from build123d import *

# Parameters (mm, degrees)
IZIM1_R                     = 27.1
Y_KSEKLIK_EKSTR_ZYON1_DEPTH = 3.3
IZIM3_R                     = 23.85
Y_KSEKLIK_EKSTR_ZYON2_DEPTH = 21.4
IZIM6_R                     = 20.35
KES_EKSTR_ZYON1_DEPTH       = 50


with BuildPart() as part:
    # Çizim1 → Yükseklik-Ekstrüzyon1 (new body)
    with BuildSketch(Plane.XY):
        Circle(IZIM1_R)
    extrude(amount=Y_KSEKLIK_EKSTR_ZYON1_DEPTH)

    # Çizim3 → Yükseklik-Ekstrüzyon2 (add)
    with BuildSketch(Plane.XY.offset(3.3)):
        Circle(IZIM3_R)
    extrude(amount=Y_KSEKLIK_EKSTR_ZYON2_DEPTH)

    # loft up to a face of the part (loft1)
    loft([Face(Wire([part.edges().sort_by_distance((-18.551226571, -19.755049803, 0))[0]])), Face(Wire([part.edges().sort_by_distance((-16.326448476, 17.385901764, 3.3))[0]]))])

    # Çizim5 → Kes-Döndür1 (revolve, cut)
    with BuildSketch(Plane(origin=(0, 0, 0), x_dir=(1, 0, 0), z_dir=(0, 1, 0))):
        Polygon((-27.1, 0), (-23.85, -3.3), (-27.1, -3.3), align=None)
    revolve(axis=Axis((0, 0, -4.734059464), (0, 0, 1)), mode=Mode.SUBTRACT)

    # Çizim6 → Kes-Ekstrüzyon1 (cut)
    with BuildSketch(Plane.XY.offset(24.7)):
        Circle(IZIM6_R)
    extrude(amount=-KES_EKSTR_ZYON1_DEPTH, mode=Mode.SUBTRACT)


solid = part.part
Design review of the part built by this model. Coordinates are the model's own, in mm. Coordinates: 2 decimals unless noted, no trailing zeros. Loops run counter-clockwise (first coordinate to the right, second up) from the corner with the lowest first, then second, coordinate; pieces in that order, holes last. Notation, with made-up numbers: (12, 81) - (59, 81) arc R19 ccw to (59, 103) - close; hole circle Ø11 at (68.25, 35.5). An arc over 180 degrees is marked (long way). Use CSV: the item, a comma, the result in double quotes. Start each with the question number.
1. Clearance check with flat-ended pins moving along their axes: pin 1 (5 mm diameter, centred on y = 10, z = 5, fed in from -X); pin 2 (8 mm diameter, centred on y = 0, z = 10.5, fed in from +X); pin 3 (3 mm diameter, centred on y = -9.5, z = 20.5, fed in from -X). State where each tip first meets the part, or that it passes through.
2. Add section A-A on y = 0. Give the boundary of the cut face in (x, z).
3. Mouldability with a two-part tool opening along X and no side actions: class faces 1 (the flat face through (3.9, 20.2, 0)), 2 (the cylindrical face through (-4.411, -19.866, 12.523)), 3 (the cylindrical face through (22.75, 7.16, 13.85)) as released by +X, released by -X, zero draft, split by the parting line, or undercut.
4. Add section C-C on z = 16. Give the boundary of the cut face in (x, y), plus the area to 3 significant figures.
5. To check wall thickness, follow probe 1 along Y at (x, z) = (0, 10); probe 2 along X at (y, z) = (-14, 9.75); probe 3 along Y at (x, z) = (-15, 23). State the ranges of each line that lie inside material, in increasing order.
Resolved:
1,pin 1,"x = -22.72"
1,pin 2,"x = 23.85"
1,pin 3,"x = -22.47"
2,outline,"(-27.1, 0) - (-20.35, 0) - (-20.35, 24.7) - (-23.85, 24.7) - (-23.85, 3.3) - close; (20.35, 0) - (27.1, 0) - (23.85, 3.3) - (23.85, 24.7) - (20.35, 24.7) - close"
3,face 1,"zero draft"
3,face 2,"undercut"
3,face 3,"split by the parting line"
4,outline,"circle Ø47.7 at (0, 0); hole circle Ø40.7 at (0, 0)"
4,area,"486 mm2"
5,probe 1,"-23.85 to -20.35, 20.35 to 23.85"
5,probe 2,"-19.31 to -14.77, 14.77 to 19.31"
5,probe 3,"-18.54 to -13.75, 13.75 to 18.54"
